from build123d import *
from build123d.topology import SkipClean

# Parameters (mm, degrees)
EXTRUDE_1_DEPTH     = 3
CUT_EXTRUDE_1_REACH = 21.647
SKETCH_3_R          = 3.25
CUT_EXTRUDE_2_DEPTH = 0.8
CUT_EXTRUDE_START   = -2.2
SKETCH_3_2_R        = 3.25
CUT_EXTRUDE_3_DEPTH = 0.8
CUT_EXTRUDE_4_DEPTH = 0.8
CUT_EXTRUDE_5_DEPTH = 0.8


with BuildPart() as part:
    # 草图1 → 凸台-拉伸1 (new body)
    with BuildSketch(Plane.XY):
        with BuildLine():
            Line((-15, -4), (15, -4))
            ThreePointArc((15, -4), (19, 0), (15, 4))
            Line((15, 4), (-15, 4))
            ThreePointArc((-15, 4), (-19, 0), (-15, -4))
        make_face()
    extrude(amount=-EXTRUDE_1_DEPTH)

    # 草图2 → 切除-拉伸1 (cut, up to next)
    with BuildSketch(Plane.XY, mode=Mode.PRIVATE) as cut_extrude_1_sk1:
        with BuildLine():
            Line((-2.883140649, -1.5), (-1.322875656, -1.5))
            ThreePointArc((-1.322875656, -1.5), (0, -2), (1.322875656, -1.5))
            Line((1.322875656, -1.5), (2.883140649, -1.5))
            ThreePointArc((2.883140649, -1.5), (3.25, 0), (2.883140649, 1.5))
            Line((2.883140649, 1.5), (1.322875656, 1.5))
            ThreePointArc((1.322875656, 1.5), (0, 2), (-1.322875656, 1.5))
            Line((-1.322875656, 1.5), (-2.883140649, 1.5))
            ThreePointArc((-2.883140649, 1.5), (-3.25, 0), (-2.883140649, -1.5))
        make_face()
    cut_extrude_1_tool1 = extrude(cut_extrude_1_sk1.sketch, amount=-CUT_EXTRUDE_1_REACH, mode=Mode.PRIVATE) & part.part
    # 草图2 → 切除-拉伸1 (cut, up to next)
    with BuildSketch(Plane.XY, mode=Mode.PRIVATE) as cut_extrude_1_sk2:
        with BuildLine():
            Line((-17.883140649, 1.5), (-16.322875656, 1.5))
            ThreePointArc((-16.322875656, 1.5), (-15, 2), (-13.677124344, 1.5))
            Line((-13.677124344, 1.5), (-12.116859351, 1.5))
            ThreePointArc((-12.116859351, 1.5), (-11.75, 0), (-12.116859351, -1.5))
            Line((-12.116859351, -1.5), (-13.677124344, -1.5))
            ThreePointArc((-13.677124344, -1.5), (-15, -2), (-16.322875656, -1.5))
            Line((-16.322875656, -1.5), (-17.883140649, -1.5))
            ThreePointArc((-17.883140649, -1.5), (-18.25, 0), (-17.883140649, 1.5))
        make_face()
    cut_extrude_1_tool2 = extrude(cut_extrude_1_sk2.sketch, amount=-CUT_EXTRUDE_1_REACH, mode=Mode.PRIVATE) & part.part
    # 草图2 → 切除-拉伸1 (cut, up to next)
    with BuildSketch(Plane.XY, mode=Mode.PRIVATE) as cut_extrude_1_sk3:
        with BuildLine():
            Line((12.116859351, 1.5), (13.677124344, 1.5))
            ThreePointArc((13.677124344, 1.5), (15, 2), (16.322875656, 1.5))
            Line((16.322875656, 1.5), (17.883140649, 1.5))
            ThreePointArc((17.883140649, 1.5), (18.25, 0), (17.883140649, -1.5))
            Line((17.883140649, -1.5), (16.322875656, -1.5))
            ThreePointArc((16.322875656, -1.5), (15, -2), (13.677124344, -1.5))
            Line((13.677124344, -1.5), (12.116859351, -1.5))
            ThreePointArc((12.116859351, -1.5), (11.75, 0), (12.116859351, 1.5))
        make_face()
    cut_extrude_1_tool3 = extrude(cut_extrude_1_sk3.sketch, amount=-CUT_EXTRUDE_1_REACH, mode=Mode.PRIVATE) & part.part
    add(cut_extrude_1_tool1.solids().sort_by_distance((0, 0, 0))[0], mode=Mode.SUBTRACT)
    add(cut_extrude_1_tool2.solids().sort_by_distance((-15, 0, 0))[0], mode=Mode.SUBTRACT)
    add(cut_extrude_1_tool3.solids().sort_by_distance((15, 0, 0))[0], mode=Mode.SUBTRACT)

    # 草图3 → 切除-拉伸2 (cut)
    with SkipClean():  # the faces are left unmerged after this step: merging them gives an invalid solid
        with BuildSketch(Plane.XY):
            with Locations((-15, 0)):
                Circle(SKETCH_3_R)
            Circle(SKETCH_3_R)
            with Locations((15, 0)):
                Circle(SKETCH_3_R)
        extrude(amount=-CUT_EXTRUDE_2_DEPTH, mode=Mode.SUBTRACT)

    # 草图3<2> → 切除-拉伸3 (cut)
    with SkipClean():  # the faces are left unmerged after this step: merging them gives an invalid solid
        with BuildSketch(Plane.XY.offset(CUT_EXTRUDE_START)):
            with Locations((-15, 0)):
                Circle(SKETCH_3_2_R)
            Circle(SKETCH_3_2_R)
            with Locations((15, 0)):
                Circle(SKETCH_3_2_R)
        extrude(amount=-CUT_EXTRUDE_3_DEPTH, mode=Mode.SUBTRACT)

    # 草图4 → 切除-拉伸4 (cut)
    with SkipClean():  # the faces are left unmerged after this step: merging them gives an invalid solid
        with BuildSketch(Plane.XY):
            with BuildLine():
                Line((-11.535898385, 2), (-3.464101615, 2))
                ThreePointArc((-3.464101615, 2), (-4, 0), (-3.464101615, -2))
                Line((-3.464101615, -2), (-11.535898385, -2))
                ThreePointArc((-11.535898385, -2), (-11, 0), (-11.535898385, 2))
            make_face()
            with BuildLine():
                Line((3.464101615, 2), (11.535898385, 2))
                ThreePointArc((11.535898385, 2), (11, 0), (11.535898385, -2))
                Line((11.535898385, -2), (3.464101615, -2))
                ThreePointArc((3.464101615, -2), (4, 0), (3.464101615, 2))
            make_face()
        extrude(amount=-CUT_EXTRUDE_4_DEPTH, mode=Mode.SUBTRACT)

    # 草图4<2> → 切除-拉伸5 (cut)
    with SkipClean():  # the faces are left unmerged after this step: merging them gives an invalid solid
        with BuildSketch(Plane.XY.offset(CUT_EXTRUDE_START)):
            with BuildLine():
                Line((-11.535898385, 2), (-3.464101615, 2))
                ThreePointArc((-3.464101615, 2), (-4, 0), (-3.464101615, -2))
                Line((-3.464101615, -2), (-11.535898385, -2))
                ThreePointArc((-11.535898385, -2), (-11, 0), (-11.535898385, 2))
            make_face()
            with BuildLine():
                Line((3.464101615, 2), (11.535898385, 2))
                ThreePointArc((11.535898385, 2), (11, 0), (11.535898385, -2))
                Line((11.535898385, -2), (3.464101615, -2))
                ThreePointArc((3.464101615, -2), (4, 0), (3.464101615, 2))
            make_face()
        extrude(amount=-CUT_EXTRUDE_5_DEPTH, mode=Mode.SUBTRACT)


solid = part.part
The model under review builds one solid part; all positions refer to its coordinate system, in mm. A direction names the side the tool comes from. Give positions to 0.01 mm unless a question says otherwise; leave off trailing zeros. Loops run counter-clockwise (first coordinate to the right, second up) from the corner with the lowest first, then second, coordinate; pieces in that order, holes last. Notation, with made-up numbers: (1.5, 67) -> (51.5, 67) arc R14 cw to (51.5, 77) -> close; hole circle Ø10 at (-8.5, 72). An arc over 180 degrees is marked (long way). Answer as a JSON object with one key per item and string values. Group by question number.
Q1. Insertion check: pin 1 (1 mm diameter, centred on y = 1.5, z = -0.5, fed in from -X); pin 2 (0.9 mm diameter, centred on x = 16.5, y = 2.5, fed in from -Z); pin 3 (0.9 mm diameter, centred on x = -14.5, y = -2.5, fed in from -Z); pin 4 (2 mm diameter, centred on x = -7, y = 0.5, fed in from +Z). Each pin has a flat end and moves straight along its axis. Give the tip position at first contact, or say it passes through.
Q2. Take a section at B-B (z = -1.8). Write out the cut boundary in (x, y).
Q3. Take a section at A-A (y = 0). State how many separate pieces and enclosed holes the cut face has, plus the area to 3 significant figures.
Q4. Tool access review of faces 4 (the flat face through (-15, 2.4, -2.2)), 5 (the flat face through (-15, -2.4, -0.8)), 6 (the flat face through (17, 1.5, -1)): name each direction out of +Z, -Z, +X, -X, +Y, -Y from which nothing blocks a thin tool from reaching the whole face with its end or side.
Q5. Wall thickness on line 1 along X through (y, z) = (1.25, -2.35); line 2 along X through (y, z) = (-0.75, -0.55); line 3 along Y through (x, z) = (5.5, -2.6): over which ranges is each line inside the solid? List them lowest first.
Q6. Draft analysis for pull direction Y (two halves, no side actions). For faces 1 (the flat face through (0, -4, -1)), 2 (the flat face through (-17, -1.5, -1)), 3 (the flat face through (-0.3, -3.5, -3)), state which applies: pulls with the +Y half, pulls with the -Y half, needs draft (parallel to the pull), parting line crosses it, or undercut.
Answer below:
{
 "1": {"pin 1": "stops at x = -18.87", "pin 2": "stops at z = -3", "pin 3": "stops at z = -2.2", "pin 4": "stops at z = -0.8"},
 "2": {"outline": "(-15, -4) -> (15, -4) arc R4 ccw to (15, 4) -> (-15, 4) arc R4 ccw to start; hole (-17.88, -1.5) -> (-16.32, -1.5) arc R2 ccw to (-13.68, -1.5) -> (-12.12, -1.5) arc R3.25 ccw to (-12.12, 1.5) -> (-13.68, 1.5) arc R2 ccw to (-16.32, 1.5) -> (-17.88, 1.5) arc R3.25 ccw to start; hole (-2.88, -1.5) -> (-1.32, -1.5) arc R2 ccw to (1.32, -1.5) -> (2.88, -1.5) arc R3.25 ccw to (2.88, 1.5) -> (1.32, 1.5) arc R2 ccw to (-1.32, 1.5) -> (-2.88, 1.5) arc R3.25 ccw to start; hole (12.12, -1.5) -> (13.68, -1.5) arc R2 ccw to (16.32, -1.5) -> (17.88, -1.5) arc R3.25 ccw to (17.88, 1.5) -> (16.32, 1.5) arc R2 ccw to (13.68, 1.5) -> (12.12, 1.5) arc R3.25 ccw to start"},
 "3": {"separate pieces": "4", "enclosed holes": "0", "area": "33.1 mm2"},
 "4": {"face 4": "-Z", "face 5": "+Z", "face 6": "+Z, -Z"},
 "5": {"line 1": "x = -18.8 to -18, -12 to -11.2, -3.8 to -3, 3 to 3.8, 11.2 to 12, 18 to 18.8", "line 2": "x = -18.93 to -18.16, -11.84 to -11.07, -3.93 to -3.16, 3.16 to 3.93, 11.07 to 11.84, 18.16 to 18.93", "line 3": "y = -4 to -2, 2 to 4"},
 "6": {"face 1": "pulls with the -Y half", "face 2": "undercut", "face 3": "needs draft"}
}
